Source: CAD feature listing. Evaluate the final solid. Frame: model axes, mm. A direction names the side the tool comes from. Round coordinates to 2 decimals unless told otherwise and drop trailing zeros. Write each loop counter-clockwise with the first axis right and the second up, starting at its lowest first coordinate (ties: lowest second). Pieces come first, ordered by that corner, then holes. Notation, with made-up numbers: (26, 44) -> (76, 44) arc R17 cw to (76, 58) -> close; hole circle Ø6 at (44.25, -35). An arc over 180 degrees is marked (long way). Return JSON: item names as keys, results as strings. Group by question number.
from build123d import *

# Parameters (mm, degrees)
SKETCH1_R           = 9.525
BOSS_EXTRUDE1_DEPTH = 6.35
EXTRUDE_THIN1_DEPTH = 88.9
SKETCH3_R           = 7.112
CUT_EXTRUDE1_DEPTH  = 144.824345992
CIRPATTERN1_COUNT   = 4


with BuildPart() as part:
    # Sketch1 → Boss-Extrude1 (new body)
    with BuildSketch(Plane.XY):
        with BuildLine():
            Line((-73.025, 76.2), (73.025, 76.2))
            ThreePointArc((73.025, 76.2), (75.27006403, 75.27006403), (76.2, 73.025))
            Line((76.2, 73.025), (76.2, -73.025))
            ThreePointArc((76.2, -73.025), (75.27006403, -75.27006403), (73.025, -76.2))
            Line((73.025, -76.2), (-73.025, -76.2))
            ThreePointArc((-73.025, -76.2), (-75.27006403, -75.27006403), (-76.2, -73.025))
            Line((-76.2, -73.025), (-76.2, 73.025))
            ThreePointArc((-76.2, 73.025), (-75.27006403, 75.27006403), (-73.025, 76.2))
        make_face()
        with Locations((-53.975, 53.975)):
            Circle(SKETCH1_R, mode=Mode.SUBTRACT)
        with Locations((-53.975, -53.975)):
            Circle(SKETCH1_R, mode=Mode.SUBTRACT)
        with Locations((53.975, 53.975)):
            Circle(SKETCH1_R, mode=Mode.SUBTRACT)
        with Locations((53.975, -53.975)):
            Circle(SKETCH1_R, mode=Mode.SUBTRACT)
    extrude(amount=BOSS_EXTRUDE1_DEPTH)

    # Sketch2 → Extrude-Thin1 (add)
    with BuildSketch(Plane.XY.offset(6.35)):
        with BuildLine():
            Line((-41.982697366, -16.388967421), (-16.388967421, -41.982697366))
            ThreePointArc((-16.388967421, -41.982697366), (-14.592916197, -42.726646142), (-12.796864973, -41.982697366))
            Line((-12.796864973, -41.982697366), (41.982697366, 12.796864973))
            ThreePointArc((41.982697366, 12.796864973), (42.726646142, 14.592916197), (41.982697366, 16.388967421))
            Line((41.982697366, 16.388967421), (16.388967421, 41.982697366))
            Line((16.388967421, 41.982697366), (20.879095481, 46.472825427))
            Line((20.879095481, 46.472825427), (46.472825427, 20.879095481))
            ThreePointArc((46.472825427, 20.879095481), (49.076646142, 14.592916197), (46.472825427, 8.306736912))
            Line((46.472825427, 8.306736912), (-8.306736912, -46.472825427))
            ThreePointArc((-8.306736912, -46.472825427), (-14.592916197, -49.076646142), (-20.879095481, -46.472825427))
            Line((-20.879095481, -46.472825427), (-46.472825427, -20.879095481))
            Line((-46.472825427, -20.879095481), (-41.982697366, -16.388967421))
        make_face()
    extrude(amount=EXTRUDE_THIN1_DEPTH)

    # Sketch3 → Cut-Extrude1 (cut, through all)
    with BuildSketch(Plane(origin=(0, 0, 0), x_dir=(-0.7071067811865511, -0.707106781186544, 0), z_dir=(0.707106781186544, -0.7071067811865511, 0))):
        with Locations((-20.6375, -30.1625)):
            Circle(SKETCH3_R)
        with Locations((-20.6375, -71.4375)):
            Circle(SKETCH3_R)
        with Locations((20.6375, -71.4375)):
            Circle(SKETCH3_R)
        with Locations((20.6375, -30.1625)):
            Circle(SKETCH3_R)
    cut_extrude1 = extrude(amount=CUT_EXTRUDE1_DEPTH, mode=Mode.SUBTRACT)

    # CirPattern1: Cut-Extrude1 ×4 about axis, 1 skipped
    cirpattern1_axis = Axis((14.592916197, 14.592916197, 71.4375), (0, 0, -1))
    add([cut_extrude1.rotate(cirpattern1_axis, i * 360 / CIRPATTERN1_COUNT) for i in range(1, CIRPATTERN1_COUNT) if i not in (2,)], mode=Mode.SUBTRACT)


solid = part.part
Item 1: Cut plane D-D on x = 11.5. Output: boundary loops of the cut face in (y, z), and give its area (3 significant figures).
Item 2: Material intervals for probe 1 along Y at (x, z) = (-15, 8.5); probe 2 along Z at (x, y) = (-63, -3); probe 3 along Y at (x, z) = (30.5, 90.5), sorted ascending.
Item 3: Pull-direction query (X, two-part tool) for faces 5 (the flat face through (33.497, 33.855, 50.178)), 6 (the flat face through (1, -76.2, 3)), 7 (the flat face through (-29.36, -29.01, 50.18)), 8 (the flat face through (-44.259, -18.665, 50.178)); classes: +X half, -X half, draft (parallel to the pull), parting line (faces both ways), or undercut.
Item 4: Cut plane A-A on z = 89. Output: boundary loops of the cut face in (x, y).
Item 5: Cut plane C-C on z = 68.5. Output: boundary loops of the cut face in (x, y), and give its area (3 significant figures).
Item 6: First-contact query: pin 1 Ø2 at (x, z) = (-29.5, 46) entering from +Y; pin 2 Ø10 at (y, z) = (19, 16.5) entering from -X; pin 3 Ø3 at (x, y) = (3, 57.5) entering from +Z; pin 4 Ø15 at (x, y) = (53.975, -53.975) entering from +Z. Flat tips, straight axial feed; report the tip coordinate or a pass-through.
Item 7: Set-up query: faces 1 (the flat face through (14.209, -14.976, 50.178)), 2 (the cylindrical face through (-14.495, -49.076, 50.178)), 3 (the flat face through (29.36, 29.01, 50.18)), 4 (the cylindrical face through (49.076, 14.691, 50.178)). Return all of +Z, -Z, +X, -X, +Y, -Y with unobstructed straight access to the full face (end or side cutting, diameter ignored); none if empty.
Item 8: Cut plane B-B on x = -49.5. Output: boundary loops of the cut face in (y, z).
Here are the results:
{
 "1": {"outline": "(-76.2, 0) -> (76.2, 0) -> (76.2, 6.35) -> (-17.69, 6.35) -> (-17.69, 95.25) -> (-26.67, 95.25) -> (-26.67, 6.35) -> (-76.2, 6.35) -> close", "area": "1,770 mm^2"},
 "2": {"probe 1": "y = -49.07 to -42.69", "probe 2": "z = 0 to 6.35", "probe 3": "y = -7.67 to 1.31, 27.87 to 36.85"},
 "3": {"face 5": "+X half", "face 6": "draft", "face 7": "undercut", "face 8": "-X half"},
 "4": {"outline": "(-46.47, -20.88) -> (-20.88, -46.47) arc R8.89 ccw to (-8.31, -46.47) -> (46.47, 8.31) arc R8.89 ccw to (46.47, 20.88) -> (20.88, 46.47) -> (16.39, 41.98) -> (41.98, 16.39) arc R2.54 cw to (41.98, 12.8) -> (-12.8, -41.98) arc R2.54 cw to (-16.39, -41.98) -> (-41.98, -16.39) -> close"},
 "5": {"outline": "(-46.47, -20.88) -> (-38.26, -29.1) -> (-33.77, -24.61) -> (-41.98, -16.39) -> close; (-29.1, -38.26) -> (-20.88, -46.47) arc R8.89 ccw to (-8.31, -46.47) -> (-0.09, -38.26) -> (-4.58, -33.77) -> (-12.8, -41.98) arc R2.54 cw to (-16.39, -41.98) -> (-24.61, -33.77) -> close; (4.58, -24.61) -> (9.07, -29.1) -> (29.1, -9.07) -> (24.61, -4.58) -> close; (16.39, 41.98) -> (24.61, 33.77) -> (29.1, 38.26) -> (20.88, 46.47) -> close; (33.77, 4.58) -> (38.26, 0.09) -> (46.47, 8.31) arc R8.89 ccw to (46.47, 20.88) -> (38.26, 29.1) -> (33.77, 24.61) -> (41.98, 16.39) arc R2.54 cw to (41.98, 12.8) -> close", "area": "737 mm^2"},
 "6": {"pin 1": "stops at y = -27.87", "pin 2": "stops at x = 34.37", "pin 3": "stops at z = 6.35", "pin 4": "passes through"},
 "7": {"face 1": "+Z", "face 2": "+Z, -Y", "face 3": "+Z, -X", "face 4": "+Z, +X"},
 "8": {"outline": "(-76.2, 0) -> (-62.38, 0) -> (-62.38, 6.35) -> (-76.2, 6.35) -> close; (-45.57, 0) -> (45.57, 0) -> (45.57, 6.35) -> (-45.57, 6.35) -> close; (62.38, 0) -> (76.2, 0) -> (76.2, 6.35) -> (62.38, 6.35) -> close"}
}
